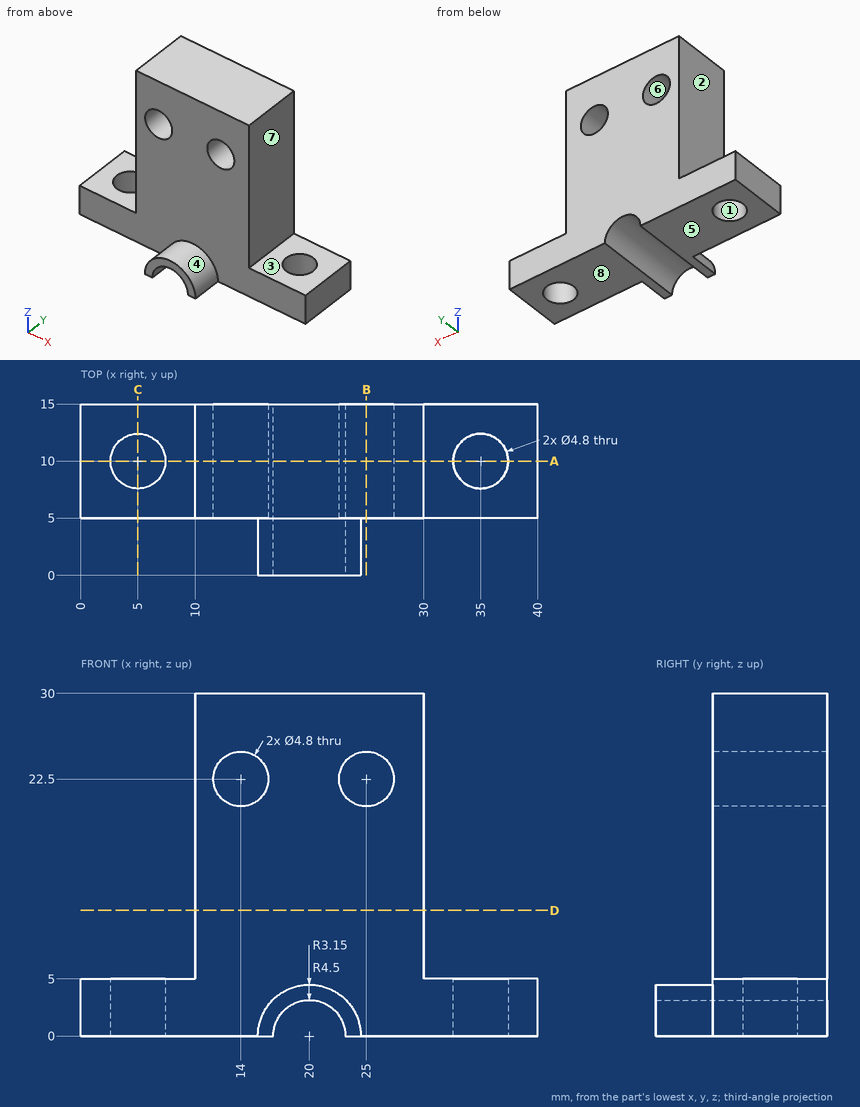
Input: dimensioned drawing with shaded views. Units: mm. Origin: part minimum x, y, z. A direction names the side the tool comes from. Give positions to 0.01 mm unless a question says otherwise; leave off trailing zeros. Order: outer loops, then holes, each group sorted by start corner. A loop starts at its lowest first (then second) coordinate and runs counter-clockwise, first axis right, second up. Notation, with made-up numbers: (-30, -20) -> (4, -20) arc R16 ccw to (4, -4) -> close; hole circle Ø5 at (-34.75, 32.5). An arc over 180 degrees is marked (long way). Use one line per item in the form item = value.
1) Section B-B, the plane x = 25. Return loops of the section in (y, z), and give its area (3 significant figures).
Response values:
outline = (5, 0) -> (15, 0) -> (15, 20.1) -> (5, 20.1) -> close; (5, 24.9) -> (15, 24.9) -> (15, 30) -> (5, 30) -> close
area = 252 mm^2
2) Section A-A, the plane y = 10. Return loops of the section in (x, z).
Response values:
outline = (0, 0) -> (2.6, 0) -> (2.6, 5) -> (0, 5) -> close; (7.4, 0) -> (16.85, 0) arc R3.15 cw to (23.15, 0) -> (32.6, 0) -> (32.6, 5) -> (30, 5) -> (30, 30) -> (10, 30) -> (10, 5) -> (7.4, 5) -> close; (37.4, 0) -> (40, 0) -> (40, 5) -> (37.4, 5) -> close; hole circle Ø4.8 at (14, 22.5); hole circle Ø4.8 at (25, 22.5)
3) Section C-C, the plane x = 5. Return loops of the section in (y, z).
Response values:
outline = (5, 0) -> (7.6, 0) -> (7.6, 5) -> (5, 5) -> close; (12.4, 0) -> (15, 0) -> (15, 5) -> (12.4, 5) -> close
4) Mould query, pull axis Z, two halves, no side actions, for the marked faces 6, 7 and 8. Classes: pulls with the +Z half, pulls with the -Z half, needs draft (parallel to the pull), parting line crosses it, or undercut.
Response values:
face_6 = undercut
face_7 = needs draft
face_8 = pulls with the -Z half
5) Section D-D, the plane z = 11. Return loops of the section in (x, y), and give its area (3 significant figures).
Response values:
outline = (10, 5) -> (30, 5) -> (30, 15) -> (10, 15) -> close
area = 200 mm^2
6) Reachability of the marked faces 1, 2, 3, 4 and 5 from +Z, -Z, +X, -X, +Y, -Y: full face, straight path, thin tool, end or side. Return the list, or none.
Response values:
face_1 = +Z, -Z
face_2 = +Z, -X, +Y, -Y
face_3 = +Z, +X, +Y, -Y
face_4 = +Z, -Y
face_5 = -Z, +X, -X, +Y, -Y
7) Line query: probe 1 along Y at (x, z) = (35, 3); probe 2 along Z at (x, y) = (25, 12); probe 3 along Z at (x, y) = (4, 13.5). Output: solid intervals per line, ascending.
Response values:
probe_1 = 5 to 7.6, 12.4 to 15
probe_2 = 0 to 20.1, 24.9 to 30
probe_3 = 0 to 5
8) First-contact query: pin 1 Ø8 at (y, z) = (11, 22.5) entering from -X; pin 2 Ø6 at (x, z) = (25, 22.5) entering from -Y; pin 3 Ø8 at (x, y) = (4, 11.5) entering from +Z; pin 4 Ø3 at (x, y) = (27.5, 3) entering from +Z. Flat tips, straight axial feed; report the tip coordinate or a pass-through.
Response values:
pin_1 = 10
pin_2 = 5
pin_3 = 5
pin_4 = through
